from build123d import *

# Parameters (mm, degrees)
BOX014_W     = 42
BOX014_H     = 6
BOX014_DEPTH = 14
BOX016_W     = 18
BOX016_H     = 27
BOX016_DEPTH = 14


with BuildPart() as cube009:
    # Box014 → Box014 (new body)
    with BuildSketch(Plane(origin=(-12, -6, 0), x_dir=(1, 0, 0), z_dir=(0, 0, 1))):
        with Locations((21, 3)):
            Rectangle(BOX014_W, BOX014_H)
    extrude(amount=BOX014_DEPTH)


with BuildPart() as fusion007006:
    # Box016 → Box016 (new body)
    with BuildSketch(Plane.XY):
        with Locations((9, 13.5)):
            Rectangle(BOX016_W, BOX016_H)
    extrude(amount=BOX016_DEPTH)

    # Fusion007006: union Cube009
    add(cube009.part)


solid = fusion007006.part
Design review of the part built by this model. Coordinates are the model's own, in mm. A direction names the side the tool comes from. Coordinates: 2 decimals unless noted, no trailing zeros. Order: outer loops, then holes, each group sorted by start corner. A loop starts at its lowest first (then second) coordinate and runs counter-clockwise, first axis right, second up. Notation, with made-up numbers: M 3,-29 L 52,-29 A19 cw 52,-12 Z; hole C 53.25,26.25 d4. An arc over 180 degrees is marked long. Use a Markdown table: item, result.
(1) Wall thickness on probe 1 along Y at (x, z) = (21.5, 5.75); probe 2 along X at (y, z) = (17, 10.5): over which ranges is each line inside the solid? List them lowest first.
Worked answers:
| item | result |
|---|---|
| probe 1 | y = -6 to 0 |
| probe 2 | x = 0 to 18 |
(2) For P1, Ø1.5, axis at x = -1.5, y = 19.5, coming from the +Z side; P2, Ø6, axis at x = 23.5, z = 8.5, coming from the +Y side; P3, Ø6, axis at y = 19.5, z = 4, coming from the -X side, all flat-tipped, find the tip position at first contact; note any pin that passes through.
Worked answers:
| item | result |
|---|---|
| P1 | passes through |
| P2 | stops at y = 0 |
| P3 | stops at x = 0 |
(3) Add section A-A (z = 6.5). Give the boundary of the cut face in (x, y), then the cut area to 3 significant figures.
Worked answers:
| item | result |
|---|---|
| outline | M -12,-6 L 30,-6 L 30,0 L 18,0 L 18,27 L 0,27 L 0,0 L -12,0 Z |
| area | 738 mm2 |
(4) Add section B-B (y = 6). Give the boundary of the cut face in (x, z), then the cut area to 3 significant figures.
Worked answers:
| item | result |
|---|---|
| outline | M 0,0 L 18,0 L 18,14 L 0,14 Z |
| area | 252 mm2 |
(5) For faces 1 (the flat face through (-12, -3, 7)), 2 (the flat face through (24, 0, 7)), 3 (the flat face through (-6, 0, 7)), list the 3-axis set-ups (+Z, -Z, +X, -X, +Y, -Y) from which the entire face can be reached by the end or side of a thin tool; tool diameter is ignored.
Worked answers:
| item | result |
|---|---|
| face 1 | +Z, -Z, -X, +Y, -Y |
| face 2 | +Z, -Z, +X, +Y |
| face 3 | +Z, -Z, -X, +Y |
(6) Add section C-C (x = -7.5). Give the boundary of the cut face in (y, z), then the cut area to 3 significant figures.
Worked answers:
| item | result |
|---|---|
| outline | M -6,0 L 0,0 L 0,14 L -6,14 Z |
| area | 84.0 mm2 |
